Input: part model. Units: mm. Frame: model coordinates. Face numbers are marked on the shaded views. A direction names the side the tool comes from. Give positions to 0.01 mm unless a question says otherwise; leave off trailing zeros. Write each loop counter-clockwise with the first axis right and the second up, starting at its lowest first coordinate (ties: lowest second). Pieces come first, ordered by that corner, then holes. Notation, with made-up numbers: (25.5, 15.25) -> (67.5, 15.25) arc R15 ccw to (67.5, 35.25) -> close; hole circle Ø10 at (66, 35). An arc over 180 degrees is marked (long way). Return JSON: item names as keys, results as strings. Group by question number.
Item 1: Section A-A, the plane y = 192. Return loops of the section in (x, z).
Item 2: Pin query (flat end, axial travel): P1, Ø2, axis at x = -28.5, z = 6, coming from the +Y side; P2, Ø6, axis at y = 100.5, z = 3.5, coming from the -X side; P3, Ø1, axis at y = 90.5, z = 4, coming from the -X side. Return the tip coordinate at first contact, or that it passes through.
Item 3: Set-up query: the marked faces 1 and 2. Return all of +Z, -Z, +X, -X, +Y, -Y with unobstructed straight access to the full face (end or side cutting, diameter ignored); none if empty.
Item 4: Section B-B, the plane x = 43.5. Return loops of the section in (y, z).
Item 5: Line query: line 1 (Z direction, x = 204, y = 86); line 2 (X direction, y = 97.5, z = 7.25); line 3 (Y direction, x = 133, z = 1.5) (3 decimals). Output: solid intervals per line, ascending. Write a range as [from, to].
from build123d import *

# Parameters (mm, degrees)
BOSS_EXTRUDE1_DEPTH = 1.5875
BOSS_EXTRUDE2_DEPTH = 215.526147
CUT_EXTRUDE1_DEPTH  = 12.7


with BuildPart() as part:
    # Sketch2 → Boss-Extrude1 (new body)
    with BuildSketch(Plane.XY):
        Polygon((0, 0), (114.3, 0), (419.1, 228.6), (-152.4, 152.4), align=None)
    extrude(amount=BOSS_EXTRUDE1_DEPTH)

    # Sketch6 → Boss-Extrude2 (add)
    with BuildSketch(Plane(origin=(-152.4, 152.4, 0), x_dir=(0, 0, -1), z_dir=(-0.7071067811865476, 0.7071067811865476, 0))):
        with BuildLine():
            Line((0, 7.5438), (0, 7.8613))
            ThreePointArc((0, 7.8613), (-0.371974388, 8.759325612), (-1.27, 9.1313))
            Line((-1.27, 9.1313), (-12.7, 9.1313))
            Line((-12.7, 9.1313), (-12.7, 7.5438))
            Line((-12.7, 7.5438), (-1.5875, 7.5438))
            Line((-1.5875, 7.5438), (-1.5875, 0))
            Line((-1.5875, 0), (0, 0))
            Line((0, 0), (0, 7.5438))
        make_face()
    extrude(amount=-BOSS_EXTRUDE2_DEPTH)

    # Sketch7 → Cut-Extrude1 (cut)
    with BuildSketch(Plane(origin=(0, 0, 0), x_dir=(-1, 0, 0), z_dir=(0, 0, -1))):
        Polygon((0, 0), (12.913608302, 0), (6.456804151, -6.456804151), align=None)
    extrude(amount=-CUT_EXTRUDE1_DEPTH, mode=Mode.SUBTRACT)


solid = part.part
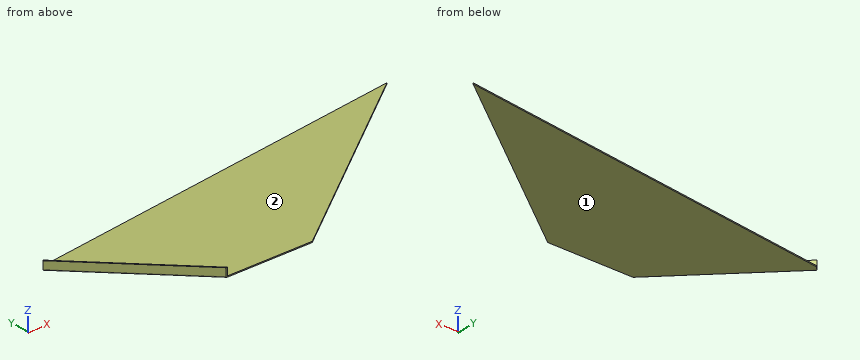
Answer below:
{
 "1": {"outline": "(144.6, 0) -> (370.3, 0) -> (370.3, 1.59) -> (144.6, 1.59) -> close"},
 "2": {"P1": "stops at y = 18.83", "P2": "stops at x = -116.41", "P3": "stops at x = -103.91"},
 "3": {"face 1": "-Z, +X, -X, +Y, -Y", "face 2": "+Z, +X, +Y"},
 "4": {"outline": "(0, 0) -> (178.52, 0) -> (178.52, 1.59) -> (0, 1.59) -> close"},
 "5": {"line 1": "z = [0, 1.59]", "line 2": "x = [-110.41, -108.17]", "line 3": "y = [14.025, 190.453]"}
}
